from build123d import *

# Parameters (mm, degrees)
F0_R     = 11.15
F1_DEPTH = 7
F2_R     = 1


with BuildPart() as f1:
    # F0 (on Top) → F1 (new body)
    with BuildSketch(Plane.XY):
        with BuildLine():
            ThreePointArc((1.3879590237, -12.9256941689), (9.6706635581, -8.6878228772), (13, 0))
            ThreePointArc((13, 0), (12.7189517514, 2.6885435362), (11.8879590237, 5.2608393105))
            ThreePointArc((11.8879590237, 5.2608393105), (11.2583302492, 6.5), (10.5, 7.6648548584))
            ThreePointArc((10.5, 7.6648548584), (0, 13), (-10.5, 7.6648548584))
            ThreePointArc((-10.5, 7.6648548584), (-11.2583302492, 6.5), (-11.8879590237, 5.2608393105))
            ThreePointArc((-11.8879590237, 5.2608393105), (-11.2583302492, -6.5), (-1.3879590237, -12.9256941689))
            ThreePointArc((-1.3879590237, -12.9256941689), (0, -13), (1.3879590237, -12.9256941689))
        make_face()
        Circle(F0_R, mode=Mode.SUBTRACT)
        with BuildLine():
            ThreePointArc((11.8879590237, 5.2608393105), (12.7189517514, 2.6885435362), (13, 0))
            ThreePointArc((13, 0), (9.6706635581, -8.6878228772), (1.3879590237, -12.9256941689))
            Line((1.3879590237, -12.9256941689), (20.7307621135, -24.0932667397))
            ThreePointArc((20.7307621135, -24.0932667397), (16.8874953738, -9.75), (31.2307621135, -5.9067332603))
            Line((31.2307621135, -5.9067332603), (11.8879590237, 5.2608393105))
        make_face()
        with BuildLine():
            ThreePointArc((-10.5, 7.6648548584), (0, 13), (10.5, 7.6648548584))
            Line((10.5, 7.6648548584), (10.5, 30))
            ThreePointArc((10.5, 30), (0, 19.5), (-10.5, 30))
            Line((-10.5, 30), (-10.5, 7.6648548584))
        make_face()
        with BuildLine():
            ThreePointArc((36.4807621135, -15), (35.0740288533, -9.75), (31.2307621135, -5.9067332603))
            ThreePointArc((31.2307621135, -5.9067332603), (16.8874953738, -9.75), (20.7307621135, -24.0932667397))
            ThreePointArc((20.7307621135, -24.0932667397), (31.2307621135, -24.0932667397), (36.4807621135, -15))
        make_face()
        Polygon((33.2337248702, -10.8125), (33.2337248702, -19.1875), (25.9807621135, -23.375), (18.7277993568, -19.1875), (18.7277993568, -10.8125), (25.9807621135, -6.625), align=None, mode=Mode.SUBTRACT)
        with BuildLine():
            Line((-20.7307621135, -24.0932667397), (-1.3879590237, -12.9256941689))
            ThreePointArc((-1.3879590237, -12.9256941689), (-11.2583302492, -6.5), (-11.8879590237, 5.2608393105))
            Line((-11.8879590237, 5.2608393105), (-31.2307621135, -5.9067332603))
            ThreePointArc((-31.2307621135, -5.9067332603), (-20.7307621135, -5.9067332603), (-15.4807621135, -15))
            ThreePointArc((-15.4807621135, -15), (-16.8874953738, -20.25), (-20.7307621135, -24.0932667397))
        make_face()
        with BuildLine():
            ThreePointArc((-10.5, 30), (0, 19.5), (10.5, 30))
            ThreePointArc((10.5, 30), (0, 40.5), (-10.5, 30))
        make_face()
        Polygon((0, 38.375), (7.2529627567, 34.1875), (7.2529627567, 25.8125), (0, 21.625), (-7.2529627567, 25.8125), (-7.2529627567, 34.1875), align=None, mode=Mode.SUBTRACT)
        with BuildLine():
            ThreePointArc((-31.2307621135, -5.9067332603), (-35.0740288533, -20.25), (-20.7307621135, -24.0932667397))
            ThreePointArc((-20.7307621135, -24.0932667397), (-16.8874953738, -20.25), (-15.4807621135, -15))
            ThreePointArc((-15.4807621135, -15), (-20.7307621135, -5.9067332603), (-31.2307621135, -5.9067332603))
        make_face()
        Polygon((-25.9807621135, -23.375), (-33.2337248702, -19.1875), (-33.2337248702, -10.8125), (-25.9807621135, -6.625), (-18.7277993568, -10.8125), (-18.7277993568, -19.1875), align=None, mode=Mode.SUBTRACT)
    extrude(amount=F1_DEPTH)

    # F2
    f2_edges = [f1.edges().sort_by_distance(p)[0] for p in [
        (-21.559361, -0.322947, 7),
        (11.059361, -18.50948, 7),
        (21.559361, -0.322947, 7),
        (10.5, 18.832427, 7),
        (-10.5, 18.832427, 7),
        (-11.059361, -18.50948, 7),
        (11.059361, -18.50948, 0),
        (-11.059361, -18.50948, 0),
        (-10.5, 18.832427, 0),
    ]]
    fillet(f2_edges, radius=F2_R)


solid = f1.part
Source: CAD feature listing. Evaluate the final solid. Frame: model axes, mm. A direction names the side the tool comes from. Round coordinates to 2 decimals unless told otherwise and drop trailing zeros. Use a Markdown table: item, result. Add a question column.
1. First-contact query: pin 1 (1 mm diameter, centred on x = 0, z = 4.5, fed in from -Y); pin 2 (2 mm diameter, centred on x = 12.5, y = 25.5, fed in from +Z); pin 3 (1 mm diameter, centred on y = -18.5, z = 4.5, fed in from +X); pin 4 (3.5 mm diameter, centred on y = 30.5, z = 5, fed in from -X). Flat tips, straight axial feed; report the tip coordinate or a pass-through.
2. Set-up query: faces 1 (the flat face through (10.92, -18.43, 3.46)), 2 (the cylindrical face through (11.34, -18.34, 6.7)), 3 (the flat face through (-18.728, -15, 3)), 4 (the cylindrical face through (-11.1, -18.2, 0.3)), 5 (the cylindrical face through (-21.55, -0.65, 0.3)). Return all of +Z, -Z, +X, -X, +Y, -Y with unobstructed straight access to the full face (end or side cutting, diameter ignored); none if empty.
3. Section query A-A (z = 5). Give the number of separate pieces and of enclosed holes in the cut face, then the cut area to 3 significant figures.
4. Mould query, pull axis Y, two halves, no side actions, for faces 6 (the flat face through (3.58, 36.31, 3.45)), 7 (the flat face through (-5.4, 10, 7)), 8 (the flat face through (7.253, 30, 3)), 9 (the cylindrical face through (0, -13, 3)). Classes: +Y half, -Y half, draft (parallel to the pull), parting line (faces both ways), or undercut.
5. Line query: probe 1 along Y at (x, z) = (-4.5, 5.25); probe 2 along X at (y, z) = (-14, 5.5); probe 3 along X at (y, z) = (16.5, 5.75). Output: solid intervals per line, ascending.
Derived:
| question | item | result |
|---|---|---|
| 1 | pin 1 | y = -13 |
| 1 | pin 2 | through |
| 1 | pin 3 | x = 36.04 |
| 1 | pin 4 | x = -10.5 |
| 2 | face 1 | +Z, -Z, -Y |
| 2 | face 2 | +Z, -Y |
| 2 | face 3 | +Z, -Z |
| 2 | face 4 | -Z, -Y |
| 2 | face 5 | -Z, -X, +Y |
| 3 | separate pieces | 1 |
| 3 | enclosed holes | 4 |
| 3 | area | 1,290 mm2 |
| 4 | face 6 | undercut |
| 4 | face 7 | draft |
| 4 | face 8 | undercut |
| 4 | face 9 | -Y half |
| 5 | probe 1 | -14.72 to -10.2, 10.2 to 24.22, 35.78 to 39.49 |
| 5 | probe 2 | -36.43 to -33.23, -18.73 to -3.25, 3.25 to 18.73, 33.23 to 36.43 |
| 5 | probe 3 | -10.5 to 10.5 |
